Verification items for the finished model (mm, model axes). A direction names the side the tool comes from. Coordinates: 2 decimals unless noted, no trailing zeros. Order: outer loops, then holes, each group sorted by start corner. A loop starts at its lowest first (then second) coordinate and runs counter-clockwise, first axis right, second up. Notation, with made-up numbers: (58.25, 0.25) -> (67.25, 0.25) arc R19 cw to (67.25, 5.25) -> close; hole circle Ø10 at (79, 1.5). An arc over 180 degrees is marked (long way). Write item = value, one per line. Start each with the question number.
from build123d import *

# Parameters (mm, degrees)
SCHIZZO2_R               = 2
TAGLIO_ESTRUSIONE1_DEPTH = 49.025821347


with BuildPart() as part:
    # Schizzo1 → Rivoluzione1 (revolve)
    with BuildSketch(Plane(origin=(0, 0, 0), x_dir=(1, 0, 0), z_dir=(0, 1, 0)), mode=Mode.PRIVATE) as rivoluzione1_sk:
        Polygon((4, 46.674184686), (8, 46.674184686), (8, 29.674184686), (7.925, 21.674184686), (7.925, 14.674184686), (4, 14.674184686), align=None)
    revolve(rivoluzione1_sk.sketch.rotate(Axis((0, 0, -88.99), (0, 0, 1)), 180), axis=Axis((0, 0, -88.99), (0, 0, 1)))

    # Schizzo2 → Taglio-Estrusione1 (cut, through all)
    with BuildSketch(Plane(origin=(0, 0, 0), x_dir=(0, 0, -1), z_dir=(1, 0, 0))):
        with Locations((18.174184686, 0)):
            Circle(SCHIZZO2_R)
    extrude(amount=-TAGLIO_ESTRUSIONE1_DEPTH, mode=Mode.SUBTRACT)


solid = part.part
Item 1: Section check B-B (y = 0). State how many separate pieces and enclosed holes the cut face has, then the cut area to 3 significant figures.
Item 2: Tool access check on faces 4 (the conical face through (-7.594, -2.392, -25.618)), 5 (the cylindrical face through (3.2, 2.4, -30.9)). Record the directions out of +Z, -Z, +X, -X, +Y, -Y that give a thin tool (end or side, any length) a straight path to the whole face; none if there is none.
Item 3: Section check A-A (z = -20.5). Record the boundary of the cut face in (x, y) (3 decimals), then the cut area to 3 significant figures.
Item 4: Gauge pin test, flat ends, axial feed: P1, Ø3, axis at y = 0, z = -18.17, coming from the -X side; P2, Ø2, axis at y = 4.5, z = -22, coming from the +X side; P3, Ø2, axis at y = 2, z = -42.5, coming from the -X side. Record the tip position at first contact, or that the pin passes through.
Item 5: Thickness scan on line 1 (Y direction, x = 0, z = -36); line 2 (Y direction, x = 1, z = -38.5). Record the ranges inside material, lowest first.
Item 6: Mould release check, pull along Y, two halves, no side actions. Record for faces 1 (the cylindrical face through (-5.66, -0.77, -20.02)), 2 (the flat face through (4, -2, -14.674)), 3 (the cylindrical face through (1.73, 7.81, -38.06)): pulls with the +Y half, pulls with the -Y half, needs draft (parallel to the pull), parting line crosses it, or undercut.
Item 7: Section check C-C (z = -26). Record the boundary of the cut face in (x, y), then the cut area to 3 significant figures.
Filled sheet:
q1.separate_pieces = 3
q1.enclosed_holes = 0
q1.area = 239 mm^2
q2.face_4 = +Z
q2.face_5 = +Z, -Z
q3.outline = circle Ø15.85 at (0, 0); hole circle Ø8 at (0, 0)
q3.area = 147 mm^2
q4.P1 = 3.71
q4.P2 = 7.11
q4.P3 = -7.94
q5.line_1 = -8 to -4, 4 to 8
q5.line_2 = -7.94 to -3.87, 3.87 to 7.94
q6.face_1 = undercut
q6.face_2 = needs draft
q6.face_3 = parting line crosses it
q7.outline = circle Ø15.93 at (0, 0); hole circle Ø8 at (0, 0)
q7.area = 149 mm^2
